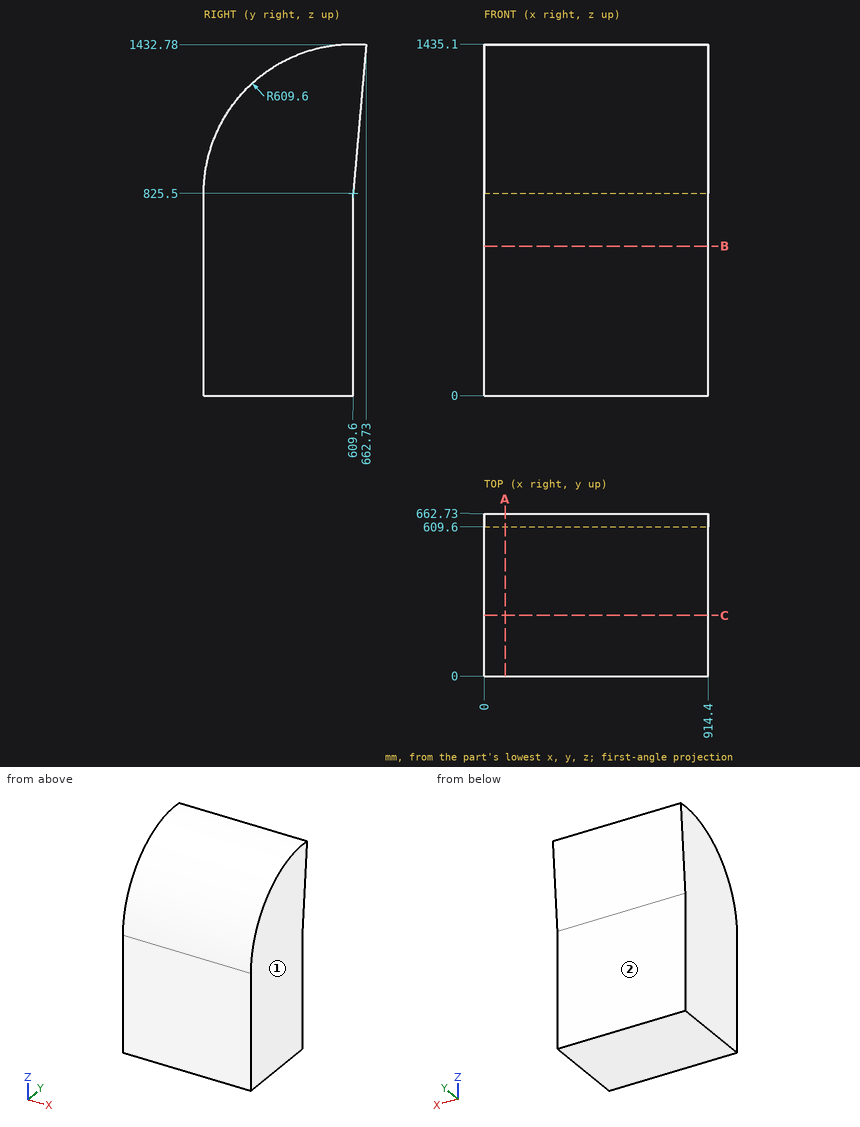
Verification items for this drawing (mm, ordinates from the low corner). A direction names the side the tool comes from. Give positions to 0.01 mm unless a question says otherwise; leave off trailing zeros. Loops run counter-clockwise (first coordinate to the right, second up) from the corner with the lowest first, then second, coordinate; pieces in that order, holes last. Notation, with made-up numbers: M 79,9.25 L 121,9.25 A17 cw 121,17.25 Z; hole C -28,43.25 d8. An arc over 180 degrees is marked long. Answer as a JSON object with one key per item and string values. Group by question number.
Item 1: Gauge pin test, flat end, axial feed: pin 1 (8 mm diameter, centred on x = 201, z = 411.5, fed in from +Y). Record the tip position at first contact, or that the pin passes through.
Item 2: Sectioned sample at B-B on z = 610. Record the boundary of the cut face in (x, y).
Item 3: Access from +Z, -Z, +X, -X, +Y, -Y to the whole of each face (thin tool, end or side, straight path). Record for the marked faces 1 and 2.
Item 4: Material ranges on L1, parallel to Y at x = 594.5, z = 100; L2, parallel to Z at x = 749.5, y = 601; L3, parallel to Z at x = 520.5, y = 496, recorded low to high.
Item 5: Sectioned sample at A-A on x = 86. Record the boundary of the cut face in (y, z), plus the area to 3 significant figures.
Item 6: Sectioned sample at C-C on y = 247. Record the boundary of the cut face in (x, z).
Findings below:
{
 "1": {"pin 1": "y = 609.6"},
 "2": {"outline": "M 0,0 L 914.4,0 L 914.4,609.6 L 0,609.6 Z"},
 "3": {"face 1": "+Z, -Z, +X, +Y, -Y", "face 2": "-Z, +X, -X, +Y"},
 "4": {"L1": "0 to 609.6", "L2": "0 to 1435.04", "L3": "0 to 1424.42"},
 "5": {"outline": "M 0,0 L 609.6,0 L 609.6,825.5 L 662.73,1432.78 A609.6 ccw 0,825.5 Z", "area": "811,000 mm2"},
 "6": {"outline": "M 0,0 L 914.4,0 L 914.4,1315.53 L 0,1315.53 Z"}
}
